Source: CAD feature listing. Evaluate the final solid. Frame: model axes, mm. Round coordinates to 2 decimals unless told otherwise and drop trailing zeros. Loops run counter-clockwise (first coordinate to the right, second up) from the corner with the lowest first, then second, coordinate; pieces in that order, holes last. Notation, with made-up numbers: (48.25, 21) - (89.25, 21) arc R31 cw to (89.25, 46) - close; hole circle Ø1 at (-38, 49.25). An arc over 180 degrees is marked (long way). One line per question, with ' | ' between items. Start each with the question number.
1. Cut plane C-C (y = 2.75). Return loops of the section in (x, z), then the cut area to 3 significant figures.
2. Pin query (flat end, axial travel): pin 1 (5.5 mm diameter, centred on x = 22.5, z = 32.5, fed in from +Y). Return the tip coordinate at first contact, or that it passes through.
3. Cut plane A-A (z = 7.5). Return loops of the section in (x, y), then the cut area to 3 significant figures.
4. Cut plane B-B (x = 0). Return loops of the section in (y, z).
5. Cut plane D-D (z = 20). Return loops of the section in (x, y).
6. Ray query, line 1 (Z direction, x = -22.5, y = 6.75); line 2 (Z direction, x = 0, y = 12.75); line 3 (X direction, y = 17, z = 5). Return the intervals inside material, ascending.
7. Mould query, pull axis X, two halves, no side actions, for faces 1 (the flat face through (0, 30, 16)), 2 (the cylindrical face through (-19.45, 14.79, 31.24)), 3 (the flat face through (30, 15, 20)). Classes: pulls with the +X half, pulls with the -X half, needs draft (parallel to the pull), parting line crosses it, or undercut.
```python
from build123d import *

# Parameters (mm, degrees)
SKETCH_W      = 60
SKETCH_H      = 40
PAD_DEPTH     = 30
SKETCH001_R   = 2.5
HOLE_DEPTH    = 30.001
SKETCH005_R   = 3.3
HOLE002_DEPTH = 30.001


with BuildPart() as part:
    # Sketch → Pad (new body)
    with BuildSketch(Plane.XZ):
        with Locations((0, 20)):
            Rectangle(SKETCH_W, SKETCH_H)
    extrude(amount=-PAD_DEPTH)

    # Sketch001 → Hole (cut, through all)
    with BuildSketch(Plane.XZ):
        with Locations((0, 20)):
            Circle(SKETCH001_R)
    extrude(amount=-HOLE_DEPTH, mode=Mode.SUBTRACT)

    # Sketch005 → Hole002 (cut, through all)
    with BuildSketch(Plane.XZ):
        with Locations((-22.5, 32.5)):
            Circle(SKETCH005_R)
        with Locations((22.5, 7.5)):
            Circle(SKETCH005_R)
        with Locations((22.5, 32.5)):
            Circle(SKETCH005_R)
        with Locations((-22.5, 7.5)):
            Circle(SKETCH005_R)
    extrude(amount=-HOLE002_DEPTH, mode=Mode.SUBTRACT)


solid = part.part
```
Answers follow:
1) outline: (-30, 0) - (30, 0) - (30, 40) - (-30, 40) - close; hole circle Ø6.6 at (-22.5, 7.5); hole circle Ø6.6 at (-22.5, 32.5); hole circle Ø5 at (0, 20); hole circle Ø6.6 at (22.5, 7.5); hole circle Ø6.6 at (22.5, 32.5) | area: 2,240 mm2
2) pin 1: passes through
3) outline: (-30, 0) - (-25.8, 0) - (-25.8, 30) - (-30, 30) - close; (-19.2, 0) - (19.2, 0) - (19.2, 30) - (-19.2, 30) - close; (25.8, 0) - (30, 0) - (30, 30) - (25.8, 30) - close | area: 1,400 mm2
4) outline: (0, 0) - (30, 0) - (30, 17.5) - (0, 17.5) - close; (0, 22.5) - (30, 22.5) - (30, 40) - (0, 40) - close
5) outline: (-30, 0) - (-2.5, 0) - (-2.5, 30) - (-30, 30) - close; (2.5, 0) - (30, 0) - (30, 30) - (2.5, 30) - close
6) line 1: z = 0 to 4.2, 10.8 to 29.2, 35.8 to 40 | line 2: z = 0 to 17.5, 22.5 to 40 | line 3: x = -30 to -24.65, -20.35 to 20.35, 24.65 to 30
7) face 1: needs draft | face 2: undercut | face 3: pulls with the +X half
